from build123d import *

# Parameters (mm, degrees)
SKETCH1_W           = 74
SKETCH1_H           = 74
SKETCH1_R           = 2.15
SKETCH1_R_2         = 19.1
SKETCH1_R_3         = 1.6
BOSS_EXTRUDE1_DEPTH = 10
SKETCH2_W           = 57.2
SKETCH2_H           = 57.2
CUT_EXTRUDE1_DEPTH  = 6
FILLET1_R           = 3
CHAMFER1_SIZE       = 1.5
FILLET2_R           = 2


with BuildPart() as part:
    # Sketch1 → Boss-Extrude1 (new body)
    with BuildSketch(Plane(origin=(0, 0, 0), x_dir=(1, 0, 0), z_dir=(0, 1, 0))):
        Rectangle(SKETCH1_W, SKETCH1_H)
        with Locations(Location((23.57, 23.57, 0), (0, 0, 270))):
            Circle(SKETCH1_R, mode=Mode.SUBTRACT)
        with Locations(Location((-23.57, 23.57, 0), (0, 0, 270))):
            Circle(SKETCH1_R, mode=Mode.SUBTRACT)
        with Locations(Location((-23.57, -23.57, 0), (0, 0, 270))):
            Circle(SKETCH1_R, mode=Mode.SUBTRACT)
        with Locations(Location((23.57, -23.57, 0), (0, 0, 270))):
            Circle(SKETCH1_R, mode=Mode.SUBTRACT)
        with Locations(Location((0, 0, 0), (0, 0, 270))):
            Circle(SKETCH1_R_2, mode=Mode.SUBTRACT)
        with Locations(Location((15.5, 31, 0), (0, 0, 270))):
            Circle(SKETCH1_R_3, mode=Mode.SUBTRACT)
        with Locations(Location((-15.5, 31, 0), (0, 0, 90))):
            Circle(SKETCH1_R_3, mode=Mode.SUBTRACT)
        with Locations(Location((31, -15.5, 0), (0, 0, 270))):
            Circle(SKETCH1_R_3, mode=Mode.SUBTRACT)
        with Locations(Location((31, 15.5, 0), (0, 0, 90))):
            Circle(SKETCH1_R_3, mode=Mode.SUBTRACT)
        with Locations(Location((-15.5, -31, 0), (0, 0, 270))):
            Circle(SKETCH1_R_3, mode=Mode.SUBTRACT)
        with Locations(Location((15.5, -31, 0), (0, 0, 90))):
            Circle(SKETCH1_R_3, mode=Mode.SUBTRACT)
        with Locations(Location((-31, 15.5, 0), (0, 0, 270))):
            Circle(SKETCH1_R_3, mode=Mode.SUBTRACT)
        with Locations(Location((-31, -15.5, 0), (0, 0, 90))):
            Circle(SKETCH1_R_3, mode=Mode.SUBTRACT)
    extrude(amount=BOSS_EXTRUDE1_DEPTH)

    # Sketch2 → Cut-Extrude1 (cut)
    with BuildSketch(Plane.XZ):
        Rectangle(SKETCH2_W, SKETCH2_H)
    extrude(amount=-CUT_EXTRUDE1_DEPTH, mode=Mode.SUBTRACT)

    # Fillet1
    fillet1_edges = [part.edges().sort_by_distance(p)[0] for p in [
        (28.6, 3, 28.6),
        (28.6, 3, -28.6),
        (-28.6, 3, -28.6),
        (-28.6, 3, 28.6),
    ]]
    fillet(fillet1_edges, radius=FILLET1_R)

    # Chamfer1
    chamfer1_edges = [part.edges().sort_by_distance(p)[0] for p in [
        (0, 10, -19.1),
        (0, 6, -19.1),
    ]]
    chamfer(chamfer1_edges, length=CHAMFER1_SIZE)

    # Fillet2
    fillet2_edges = [part.edges().sort_by_distance(p)[0] for p in [
        (37, 5, 37),
        (-37, 5, 37),
        (-37, 5, -37),
        (37, 5, -37),
    ]]
    fillet(fillet2_edges, radius=FILLET2_R)


solid = part.part
Part model, mm, in its own coordinate system. A direction names the side the tool comes from. Coordinates: 2 decimals unless noted, no trailing zeros. Order: outer loops, then holes, each group sorted by start corner. A loop starts at its lowest first (then second) coordinate and runs counter-clockwise, first axis right, second up. Notation, with made-up numbers: M 20.25,7.5 L 71.25,7.5 A8 cw 71.25,12.5 Z; hole C -11.75,53 d5. An arc over 180 degrees is marked long. One line per question, with ' | ' between items.
Q1. Pin check, flat tips, straight feed: P1, Ø17, axis at x = -14, z = -10, coming from the -Y side; P2, Ø3, axis at x = -15.5, z = -31, coming from the +Y side. Stop position of each tip, or through.
A:
P1: stops at y = 6 | P2: passes through
Q2. Slice it at A-A (z = 0). Give the cut face in (x, y), and give its area (4 significant figures).
A:
outline: M -37,0 L -28.6,0 L -28.6,6 L -20.6,6 L -19.1,7.5 L -19.1,8.5 L -20.6,10 L -37,10 Z; M 19.1,7.5 L 20.6,6 L 28.6,6 L 28.6,0 L 37,0 L 37,10 L 20.6,10 L 19.1,8.5 Z | area: 239.5 mm^2
Q3. 3-axis set-ups, long thin cutter, end or side, ignore diameter. For faces 4 (the face through (-28.6, 3, 0)), 5 (the face through (-36.43, 5.07, 36.4)): which of +Z, -Z, +X, -X, +Y, -Y reach the whole face in a straight line?
A:
face 4: -Y | face 5: +Z, -X, +Y, -Y
Q4. Two-plate mould, pull along Z, no slides. Class faces 1 (the face through (-17, 10, -17)), 2 (the face through (23.66, 7.97, 21.42)), 3 (the face through (0, 5, 37)): +Z half, -Z half, draft (parallel to the pull), parting line (faces both ways), or undercut.
A:
face 1: draft | face 2: undercut | face 3: +Z half
Q5. Slice it at B-B (x = 31). Give the cut face in (y, z), and give its area (3 significant figures).
A:
outline: M 0,-37 L 10,-37 L 10,-17.1 L 0,-17.1 Z; M 0,-13.9 L 10,-13.9 L 10,13.9 L 0,13.9 Z; M 0,17.1 L 10,17.1 L 10,37 L 0,37 Z | area: 676 mm^2
Q6. Slice it at D-D (z = 23.57). Give the cut face in (x, y).
A:
outline: M -37,0 L -28.6,0 L -28.6,6 L -25.72,6 L -25.72,10 L -37,10 Z; M -21.42,6 L 21.42,6 L 21.42,10 L -21.42,10 Z; M 25.72,6 L 28.6,6 L 28.6,0 L 37,0 L 37,10 L 25.72,10 Z
Q7. Drill centre lines: line 1 (X direction, y = 6.75, z = -31); line 2 (Z direction, x = 23.57, y = 7.1); line 3 (X direction, y = 3.5, z = 30.5). Where is each one in solid material? Low to high.
A:
line 1: x = -37 to -17.1, -13.9 to 13.9, 17.1 to 37 | line 2: z = -37 to -25.72, -21.42 to 21.42, 25.72 to 37 | line 3: x = -37 to -17.02, -13.98 to 13.98, 17.02 to 37
Q8. Slice it at C-C (y = 5). Count the separate pieces of the cut face and the enclosed holes in it, and give its area (3 significant figures).
A:
separate pieces: 1 | enclosed holes: 9 | area: 2,140 mm^2
